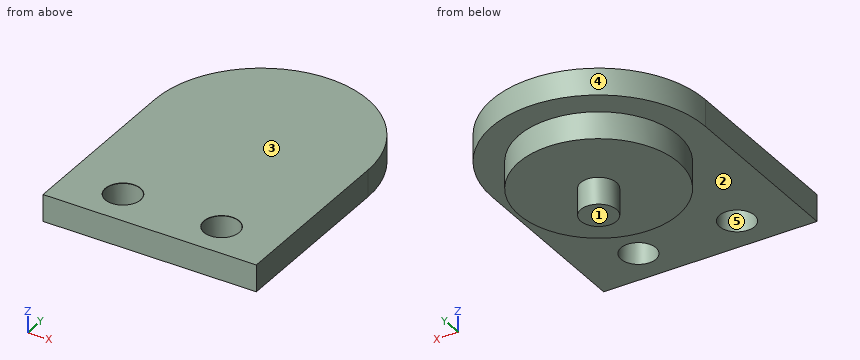
from build123d import *

# Parameters (mm, degrees)
BOSS_EXTRUDE1_DEPTH             = 3
SKETCH2_R                       = 8.9
BOSS_EXTRUDE2_DEPTH             = 3
SKETCH3_R                       = 2
BOSS_EXTRUDE3_DEPTH             = 3
M3_5_CLEARANCE_HOLE1_AT_2_COUNT = 2
M3_5_CLEARANCE_HOLE1_AT_2_PITCH = 11
M3_5_CLEARANCE_HOLE1_AT_3_COUNT = 2
M3_5_CLEARANCE_HOLE1_AT_3_PITCH = 11


with BuildPart() as part:
    # Sketch1 → Boss-Extrude1 (new body)
    with BuildSketch(Plane.XY):
        with BuildLine():
            Line((-11.9, 0), (-11.9, -20))
            Line((-11.9, -20), (11.9, -20))
            Line((11.9, -20), (11.9, 0))
            ThreePointArc((11.9, 0), (0, 11.9), (-11.9, 0))
        make_face()
    extrude(amount=BOSS_EXTRUDE1_DEPTH)

    # Sketch2 → Boss-Extrude2 (add)
    with BuildSketch(Plane(origin=(0, 0, 0), x_dir=(-1, 0, 0), z_dir=(0, 0, -1))):
        Circle(SKETCH2_R)
    extrude(amount=BOSS_EXTRUDE2_DEPTH)

    # Sketch3 → Boss-Extrude3 (add)
    with BuildSketch(Plane(origin=(0, 0, -3), x_dir=(-1, 0, 0), z_dir=(0, 0, -1))):
        Circle(SKETCH3_R)
    extrude(amount=BOSS_EXTRUDE3_DEPTH)

    # Sketch5 → M3.5 Clearance Hole1 (revolve, cut)
    with BuildSketch(Plane(origin=(-5.515156433, -15.92620122, 3), x_dir=(0, -1, 0), z_dir=(1, 0, 0))):
        Polygon((0, 0), (0, 9), (1.95, 9), (1.95, 0.025), (1.975, 0), align=None)
    m3_5_clearance_hole1 = revolve(axis=Axis((-5.515156433, -15.92620122, 9.35), (0, 0, -1)), mode=Mode.SUBTRACT)

    # M3.5 Clearance Hole1 at 2: M3.5 Clearance Hole1 ×2
    with Locations(*[(i * M3_5_CLEARANCE_HOLE1_AT_2_PITCH, 0, 0) for i in range(1, M3_5_CLEARANCE_HOLE1_AT_2_COUNT)]):
        add(m3_5_clearance_hole1, mode=Mode.SUBTRACT)

    # M3.5 Clearance Hole1 at 3: M3.5 Clearance Hole1 ×2
    with Locations(*[(i * M3_5_CLEARANCE_HOLE1_AT_3_PITCH, 0, 0) for i in range(1, M3_5_CLEARANCE_HOLE1_AT_3_COUNT)]):
        add(m3_5_clearance_hole1, mode=Mode.SUBTRACT)


solid = part.part
Part model, mm, in its own coordinate system. Face numbers are marked on the shaded views. A direction names the side the tool comes from. Give positions to 0.01 mm unless a question says otherwise; leave off trailing zeros. Loops run counter-clockwise (first coordinate to the right, second up) from the corner with the lowest first, then second, coordinate; pieces in that order, holes last. Notation, with made-up numbers: (-36.75, 8) -> (10.25, 8) arc R19 ccw to (10.25, 41) -> close; hole circle Ø5 at (46, 57.25). An arc over 180 degrees is marked (long way). Write each question's results on one line, items separated by ' | '. Start each with the question number.
Q1. Band-saw the part on D-D on z = -3.5. List the corners of the cut face in (x, y), plus the area to 3 significant figures.
Q2. Which spindle directions (+Z, -Z, +X, -X, +Y, -Y) get a long thin tool onto all of the face, cutting with end or side? Do the marked faces 1 and 2. Say none if no direction does.
Q3. Wall check: L1, parallel to X at y = -14.5, z = 0.25; L2, parallel to Z at x = -9.75, y = -7.5; L3, parallel to Z at x = 3, y = -7. Give the ranges that are in metal, low to high.
Q4. Pull direction X, two halves, no side cores. Call the marked faces 3, 4 and 5: +X half, -X half, draft (parallel to the pull), parting line (faces both ways), or undercut.
Q5. Band-saw the part on A-A on x = 0. List the corners of the cut face in (y, z).
Q6. Pin check, flat tips, straight feed: P1, Ø3, axis at x = 6.5, y = -16, coming from the -Z side; P2, Ø3, axis at y = 2, z = 0, coming from the -X side; P3, Ø5, axis at x = -3, z = 0.5, coming from the +Y side; P4, Ø2, axis at y = -11.5, z = -3.5, coming from the -X side. Stop position of each tip, or through.
Q7. Band-saw the part on C-C on y = 8.5. List the corners of the cut face in (x, z).
Q8. Band-saw the part on B-B on z = 2. List the corners of the cut face in (x, y).
Results are:
1) outline: circle Ø4 at (0, 0) | area: 12.6 mm²
2) face 1: -Z, +X, -X, +Y, -Y | face 2: -Z
3) L1: x = -11.9 to -6.84, -4.19 to 4.16, 6.81 to 11.9 | L2: z = 0 to 3 | L3: z = -3 to 3
4) face 3: draft | face 4: parting line | face 5: undercut
5) outline: (-20, 0) -> (-8.9, 0) -> (-8.9, -3) -> (-2, -3) -> (-2, -6) -> (2, -6) -> (2, -3) -> (8.9, -3) -> (8.9, 0) -> (11.9, 0) -> (11.9, 3) -> (-20, 3) -> close
6) P1: stops at z = 0 | P2: stops at x = -11.89 | P3: stops at y = 11.89 | P4: passes through
7) outline: (-8.33, 0) -> (-2.64, 0) -> (-2.64, -3) -> (2.64, -3) -> (2.64, 0) -> (8.33, 0) -> (8.33, 3) -> (-8.33, 3) -> close
8) outline: (-11.9, -20) -> (11.9, -20) -> (11.9, 0) arc R11.9 ccw to (-11.9, 0) -> close; hole circle Ø3.9 at (-5.52, -15.93); hole circle Ø3.9 at (5.48, -15.93)
